Model file for the job. Use its own axes, mm. A direction names the side the tool comes from. Round coordinates to 2 decimals unless told otherwise and drop trailing zeros. Loops run counter-clockwise (first coordinate to the right, second up) from the corner with the lowest first, then second, coordinate; pieces in that order, holes last. Notation, with made-up numbers: (62.5, 75) -> (83.5, 75) arc R24 ccw to (83.5, 107) -> close; hole circle Ø2 at (7, 69.25). An arc over 180 degrees is marked (long way). Use a Markdown table: item, result.
from build123d import *

# Parameters (mm, degrees)
SKETCH1_W            = 450.85
SKETCH1_H            = 101.6
BOSS_EXTRUDE1_DEPTH  = 19.05
SKETCH2_R            = 3.175
CUT_EXTRUDE1_DEPTH   = 455.102703141
CONVERT_SOLID2_START = -50.8
CONVERT_SOLID2_DEPTH = 101.6


# Read off the part's stored shape, not the designer's step: Convert-Solid2
with BuildPart() as part:
    # Sketch1 → Boss-Extrude1 (new body)
    with BuildSketch(Plane(origin=(0, 0, 0), x_dir=(1, 0, 0), z_dir=(0, 1, 0))):
        Rectangle(SKETCH1_W, SKETCH1_H)
    extrude(amount=BOSS_EXTRUDE1_DEPTH)

    # Sketch2 → Cut-Extrude1 (cut, through all)
    with BuildSketch(Plane(origin=(225.425, 0, 0), x_dir=(0, 0, -1), z_dir=(1, 0, 0))):
        with Locations((-38.1, 6.35)):
            Circle(SKETCH2_R)
        with Locations((-19.05, 6.35)):
            Circle(SKETCH2_R)
        with Locations((0, 6.35)):
            Circle(SKETCH2_R)
        with Locations((19.05, 6.35)):
            Circle(SKETCH2_R)
    extrude(amount=-CUT_EXTRUDE1_DEPTH, mode=Mode.SUBTRACT)

    # Convert-Solid2 outline → Convert-Solid2 (cut)
    with BuildSketch(Plane.XY.offset(CONVERT_SOLID2_START)):
        with BuildLine():
            ThreePointArc((219.075, 19.05), (223.565128061, 17.190128061), (225.425, 12.7))
            Line((225.425, 12.7), (225.425, 19.05))
            Line((225.425, 19.05), (219.075, 19.05))
        make_face()
        with BuildLine():
            ThreePointArc((-225.425, 12.7), (-223.565128061, 17.190128061), (-219.075, 19.05))
            Line((-219.075, 19.05), (-225.425, 19.05))
            Line((-225.425, 19.05), (-225.425, 12.7))
        make_face()
        with BuildLine():
            Line((-222.25, 0), (222.25, 0))
            Line((222.25, 0), (222.25, 12.7))
            ThreePointArc((222.25, 12.7), (221.32006403, 14.94506403), (219.075, 15.875))
            Line((219.075, 15.875), (-219.075, 15.875))
            ThreePointArc((-219.075, 15.875), (-221.32006403, 14.94506403), (-222.25, 12.7))
            Line((-222.25, 12.7), (-222.25, 0))
        make_face()
    extrude(amount=CONVERT_SOLID2_DEPTH, mode=Mode.SUBTRACT)


solid = part.part
Q1. Flat gauge pins, fed straight in: pin 1 (7.5 mm diameter, centred on y = 6.35, z = -19.05, fed in from +X) (3 decimals); pin 2 (1 mm diameter, centred on y = 15, z = 16.5, fed in from +X); pin 3 (4 mm diameter, centred on y = 16, z = -5, fed in from +X). Where does each tip first touch, or does it go through?
Results list:
| item | result |
|---|---|
| pin 1 | stops at x = 225.425 |
| pin 2 | stops at x = 225.16 |
| pin 3 | stops at x = 225.29 |
Q2. Band-saw the part on B-B, the plane x = -120. Give the cut face in (y, z) (3 decimals).
Results list:
| item | result |
|---|---|
| outline | (15.875, -50.8) -> (19.05, -50.8) -> (19.05, 50.8) -> (15.875, 50.8) -> close |
Q3. Tool access for faces 1 (the face through (-222.25, 11, -1)), 2 (the face through (-1, 17, -50.8)): list every direction of +Z, -Z, +X, -X, +Y, -Y with a clear straight run to the whole face (end or side of a thin tool).
Results list:
| item | result |
|---|---|
| face 1 | +Z, -Z, -Y |
| face 2 | -Z, +X, -X, +Y, -Y |
Q4. Pull direction X, two halves, no side cores. Call faces 3 (the face through (-3, 19.05, -1)), 4 (the face through (225.425, 2, 1)), 5 (the face through (222.25, 2, -1)), 6 (the face through (-225.425, 2, 1)): released by +X, released by -X, zero draft, split by the parting line, or undercut.
Results list:
| item | result |
|---|---|
| face 3 | zero draft |
| face 4 | released by +X |
| face 5 | undercut |
| face 6 | released by -X |
Q5. Band-saw the part on A-A, the plane y = 6.35. Give the number of separate pieces and of enclosed holes in the cut face, plus the area to 3 significant figures.
Results list:
| item | result |
|---|---|
| separate pieces | 10 |
| enclosed holes | 0 |
| area | 484 mm² |
Q6. Drill centre lines: L1, parallel to X at y = 1.25, z = -23 (3 decimals); L2, parallel to Y at x = 109.5, z = 31 (3 decimals); L3, parallel to X at y = 14.75, z = 9.5 (3 decimals). Where is each one in solid material? Low to high. Write a range as from..to.
Results list:
| item | result |
|---|---|
| L1 | x = -225.425..-222.25, 222.25..225.425 |
| L2 | y = 15.875..19.05 |
| L3 | x = -225.085..-221.499, 221.499..225.085 |
